For this review, take the finished solid that the model builds, in its own axes (mm). Face numbers are marked on the shaded views. A direction names the side the tool comes from. Coordinates: 2 decimals unless noted, no trailing zeros. Write each loop counter-clockwise with the first axis right and the second up, starting at its lowest first coordinate (ties: lowest second). Pieces come first, ordered by that corner, then holes. Notation, with made-up numbers: (64.25, 70.5) - (81.25, 70.5) arc R8 ccw to (81.25, 76.5) - close; hole circle Ø10 at (-37.75, -22.75). An arc over 180 degrees is marked (long way). Write each question's results on one line, items separated by ' | '.
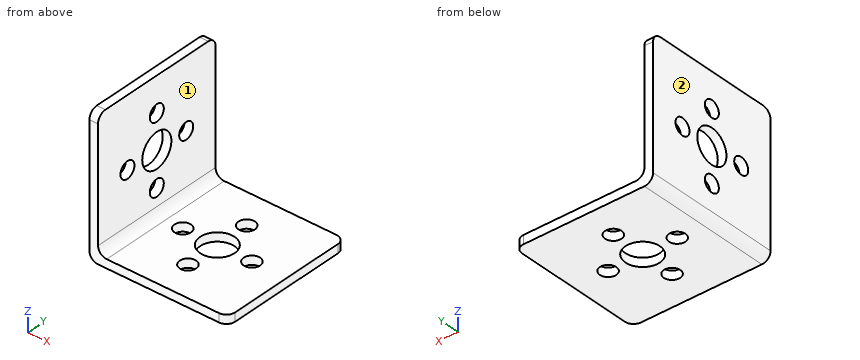
from build123d import *

# Parameters (mm, degrees)
F0_W     = 32
F0_H     = 32
F0_R     = 1.905
F0_R_2   = 3.96875
F1_DEPTH = 2
F2_W     = 2
F2_H     = 32
F3_DEPTH = 30
F4_R     = 3.96875
F4_R_2   = 1.905
F5_DEPTH = 2
F6_R     = 2


# Not quite as in the source:
# - a feature names something its author has since deleted; it is built from what else it names


with BuildPart() as f1:
    # F0 (on Top) → F1 (new body)
    with BuildSketch(Plane.XY):
        with Locations((-16, 16)):
            Rectangle(F0_W, F0_H)
        with Locations((-16, 8)):
            Circle(F0_R, mode=Mode.SUBTRACT)
        with Locations((-24, 16)):
            Circle(F0_R, mode=Mode.SUBTRACT)
        with Locations((-16, 16)):
            Circle(F0_R_2, mode=Mode.SUBTRACT)
        with Locations((-8, 16)):
            Circle(F0_R, mode=Mode.SUBTRACT)
        with Locations((-16, 24)):
            Circle(F0_R, mode=Mode.SUBTRACT)
    extrude(amount=F1_DEPTH)

    # F2 (on face) → F3 (join)
    with BuildSketch(Plane.XY.offset(2)):
        with Locations((-31, 16)):
            Rectangle(F2_W, F2_H)
    extrude(amount=F3_DEPTH)

    # F4 (on face) → F5 (cut, through all)
    with BuildSketch(Plane(origin=(-32, 0, 0), x_dir=(0, -1, 0), z_dir=(-1, 0, 0))):
        with Locations((-16, 16)):
            Circle(F4_R)
        with Locations((-16, 24)):
            Circle(F4_R_2)
        with Locations((-24, 16)):
            Circle(F4_R_2)
        with Locations((-16, 8)):
            Circle(F4_R_2)
        with Locations((-8, 16)):
            Circle(F4_R_2)
    extrude(amount=-F5_DEPTH, mode=Mode.SUBTRACT)

    # F6
    f6_edges = [f1.edges().sort_by_distance(p)[0] for p in [
        (-31, 0, 32),
        (-31, 32, 32),
        (0, 0, 1),
        (0, 32, 1),
        (-30, 16, 2),
        (-32, 16, 0),
    ]]
    fillet(f6_edges, radius=F6_R)


solid = f1.part
Q1. Take a section at D-D on x = -16.5. State the section outline as (y, z) points, plus the area to 3 significant figures.
Results found:
outline: (0, 0) - (6.16, 0) - (6.16, 2) - (0, 2) - close; (9.84, 0) - (12.06, 0) - (12.06, 2) - (9.84, 2) - close; (19.94, 0) - (22.16, 0) - (22.16, 2) - (19.94, 2) - close; (25.84, 0) - (32, 0) - (32, 2) - (25.84, 2) - close | area: 33.5 mm2
Q2. Take a section at C-C on z = 8. State the section outline as (x, y) points (3 decimals).
Results found:
outline: (-32, 0) - (-30, 0) - (-30, 14.095) - (-32, 14.095) - close; (-32, 17.905) - (-30, 17.905) - (-30, 32) - (-32, 32) - close
Q3. For the marked faces 1 and 2, list the 3-axis set-ups (+Z, -Z, +X, -X, +Y, -Y) from which the entire face can be reached by the end or side of a thin tool; tool diameter is ignored.
Results found:
face 1: +Z, +X, +Y, -Y | face 2: +Z, -Z, -X, +Y, -Y
Q4. Take a section at A-A on x = -24. State the section outline as (y, z) points (3 decimals).
Results found:
outline: (0, 0) - (14.095, 0) - (14.095, 2) - (0, 2) - close; (17.905, 0) - (32, 0) - (32, 2) - (17.905, 2) - close
Q5. Wall thickness on line 1 along Z through (x, y) = (-30.95, 16) (3 decimals); line 2 along Z through (x, y) = (-24.5, 18); line 3 along X through (y, z) = (7, 13): over which ranges is each line inside the solid? List them lowest first. Write a range as from..to.
Results found:
line 1: 0.24..6.095, 9.905..12.031, 19.969..22.095, 25.905..32 | line 2: 0..2 | line 3: -32..-30
Q6. For pin 1 (3 mm diameter, centred on y = 8, z = 16, fed in from -X); pin 2 (8.5 mm diameter, centred on y = 20.5, z = 20.5, fed in from +X); pin 3 (6 mm diameter, centred on x = -16, y = 8, fed in from +Z), all flat-tipped, find the tip position at first contact; note any pin that passes through.
Results found:
pin 1: through | pin 2: x = -30 | pin 3: z = 2
Q7. Take a section at B-B on y = 8. State the section outline as (x, z) points (3 decimals).
Results found:
outline: (-32, 2) arc R2 ccw to (-30, 0) - (-17.905, 0) - (-17.905, 2) - (-28, 2) arc R2 cw to (-30, 4) - (-30, 14.095) - (-32, 14.095) - close; (-32, 17.905) - (-30, 17.905) - (-30, 32) - (-32, 32) - close; (-14.095, 0) - (0, 0) - (0, 2) - (-14.095, 2) - close
